CAD build for the part. Positions are in the model's coordinates, mm. Face numbers are marked on the shaded views. A direction names the side the tool comes from. Give positions to 0.01 mm unless a question says otherwise; leave off trailing zeros. Loops run counter-clockwise (first coordinate to the right, second up) from the corner with the lowest first, then second, coordinate; pieces in that order, holes last. Notation, with made-up numbers: M 64.25,27.5 L 107.25,27.5 A17 ccw 107.25,60.5 Z; hole C 8.5,16 d2. An arc over 180 degrees is marked long. Answer as CSV lines item,"result".
```python
from build123d import *

# Parameters (mm, degrees)
SKETCH1_W           = 25
SKETCH1_H           = 7
SKETCH1_R           = 1.5
BOSS_EXTRUDE1_DEPTH = 3
SKETCH2_W           = 4.5
SKETCH2_H           = 7
BOSS_EXTRUDE2_DEPTH = 11
CHAMFER1_SIZE       = 1


with BuildPart() as part:
    # Sketch1 → Boss-Extrude1 (new body)
    with BuildSketch(Plane(origin=(0, 0, 0), x_dir=(1, 0, 0), z_dir=(0, 1, 0))):
        Rectangle(SKETCH1_W, SKETCH1_H)
        with Locations(Location((9, 0, 0), (0, 0, 270))):
            Circle(SKETCH1_R, mode=Mode.SUBTRACT)
        with Locations(Location((-9, 0, 0), (0, 0, 90))):
            Circle(SKETCH1_R, mode=Mode.SUBTRACT)
    extrude(amount=BOSS_EXTRUDE1_DEPTH)

    # Sketch2 → Boss-Extrude2 (add)
    with BuildSketch(Plane.XZ):
        with Locations((-3.9, 0)):
            Rectangle(SKETCH2_W, SKETCH2_H)
        with Locations((3.9, 0)):
            Rectangle(SKETCH2_W, SKETCH2_H)
    extrude(amount=-BOSS_EXTRUDE2_DEPTH)

    # Chamfer1
    chamfer1_edges = [part.edges().sort_by_distance(p)[0] for p in [
        (6.15, 11, 0),
    ]]
    chamfer(chamfer1_edges, length=CHAMFER1_SIZE)


solid = part.part
```
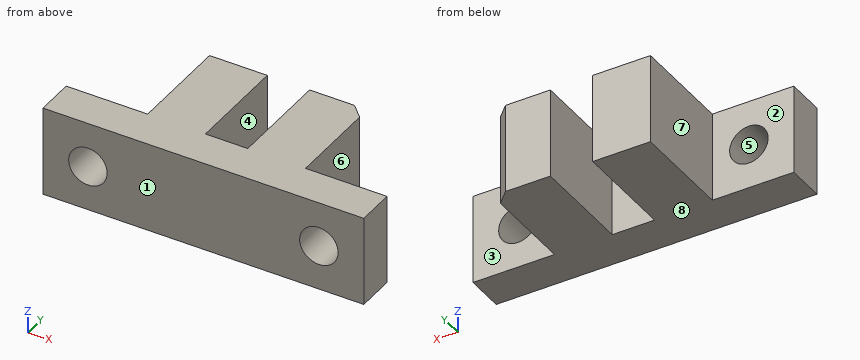
Q1. Cut at A-A (z = 0). Write the cut outline in (x, y), and give its area (4 significant figures).
Solution:
outline,"M -12.5,0 L -10.5,0 L -10.5,3 L -12.5,3 Z; M -7.5,0 L 7.5,0 L 7.5,3 L 6.15,3 L 6.15,10 L 5.15,11 L 1.65,11 L 1.65,3 L -1.65,3 L -1.65,11 L -6.15,11 L -6.15,3 L -7.5,3 Z; M 10.5,0 L 12.5,0 L 12.5,3 L 10.5,3 Z"
area,"128.5 mm²"
Q2. Which spindle directions (+Z, -Z, +X, -X, +Y, -Y) get a long thin tool onto all of the face, cutting with end or side? Do the marked faces 1, 2, 3 and 4. Say none if no direction does.
Solution:
face 1,"+Z, -Z, +X, -X, -Y"
face 2,"+Z, -Z, -X, +Y"
face 3,"+Z, -Z, +X, +Y"
face 4,"+Z, -Z, +Y"
Q3. Pin check, flat tips, straight feed: P1, Ø2, axis at y = 5.5, z = 1.5, coming from the +X side; P2, Ø1, axis at y = 10, z = 1.5, coming from the -X side; P3, Ø1.6, axis at x = 0, z = -1.5, coming from the +Y side. Stop position of each tip, or through.
Solution:
P1,"stops at x = 6.15"
P2,"stops at x = -6.15"
P3,"stops at y = 3"
Q4. Wall check: line 1 (X direction, y = 1.25, z = 0); line 2 (X direction, y = 5.25, z = 2.25); line 3 (X direction, y = 2.5, z = 1). Give the ranges that are in metal, low to high. Write a range as [from, to].
Solution:
line 1,"x = [-12.5, -10.5], [-7.5, 7.5], [10.5, 12.5]"
line 2,"x = [-6.15, -1.65], [1.65, 6.15]"
line 3,"x = [-12.5, -10.12], [-7.88, 7.88], [10.12, 12.5]"
Q5. Cut at D-D (z = -1.75). Write the cut outline in (x, y).
Solution:
outline,"M -12.5,0 L 12.5,0 L 12.5,3 L 6.15,3 L 6.15,10 L 5.15,11 L 1.65,11 L 1.65,3 L -1.65,3 L -1.65,11 L -6.15,11 L -6.15,3 L -12.5,3 Z"
Q6. Cut at B-B (x = 9). Write the cut outline in (y, z).
Solution:
outline,"M 0,-3.5 L 3,-3.5 L 3,-1.5 L 0,-1.5 Z; M 0,1.5 L 3,1.5 L 3,3.5 L 0,3.5 Z"
Q7. Cut at C-C (y = 9.5). Write the cut outline in (x, z), and give its area (3 significant figures).
Solution:
outline,"M -6.15,-3.5 L -1.65,-3.5 L -1.65,3.5 L -6.15,3.5 Z; M 1.65,-3.5 L 6.15,-3.5 L 6.15,3.5 L 1.65,3.5 Z"
area,"63.0 mm²"
Q8. Mould opens along X. For the marked faces 5, 6, 7 and 8 say: released by +X, released by -X, zero draft, split by the parting line, or undercut.
Solution:
face 5,"undercut"
face 6,"released by +X"
face 7,"released by -X"
face 8,"zero draft"
